Drawing for the job (mm, zero at the part's lowest x, y, z). A direction names the side the tool comes from. Give positions to 0.01 mm unless a question says otherwise; leave off trailing zeros. Loops run counter-clockwise (first coordinate to the right, second up) from the corner with the lowest first, then second, coordinate; pieces in that order, holes last.
1) Flat gauge pins, fed straight in: P1, Ø5.5, axis at x = 63.5, y = 24.003, coming from the +Z side (3 decimals); P2, Ø11.5, axis at x = 34.925, y = 16.002, coming from the +Z side; P3, Ø5, axis at x = 31.5, y = 18.5, coming from the -Z side; P4, Ø7.5, axis at x = 23.5, z = 8.5, coming from the +Y side (3 decimals). Where does each tip first touch, or does it go through?
2) Band-saw the part on D-D on x = 58.5. List the corners of the cut face in (y, z) (3 decimals).
3) Band-saw the part on C-C on y = 41. List the corners of the cut face in (x, z) (3 decimals), then the cut area to 3 significant figures.
4) 3-axis set-ups, long thin cutter, end or side, ignore diameter. For the marked faces 1 and 2: which of +Z, -Z, +X, -X, +Y, -Y reach the whole face in a straight line?
5) Band-saw the part on A-A on x = 6.35. List the corners of the cut face in (y, z) (3 decimals).
6) Band-saw the part on B-B on z = 6.35. List the corners of the cut face in (x, y) (3 decimals).
7) Wall check: line 1 (Y direction, x = 63.5, z = 2); line 2 (Y direction, x = 35, z = 11.5) (3 decimals). Give the ranges that are in metal, low to high.
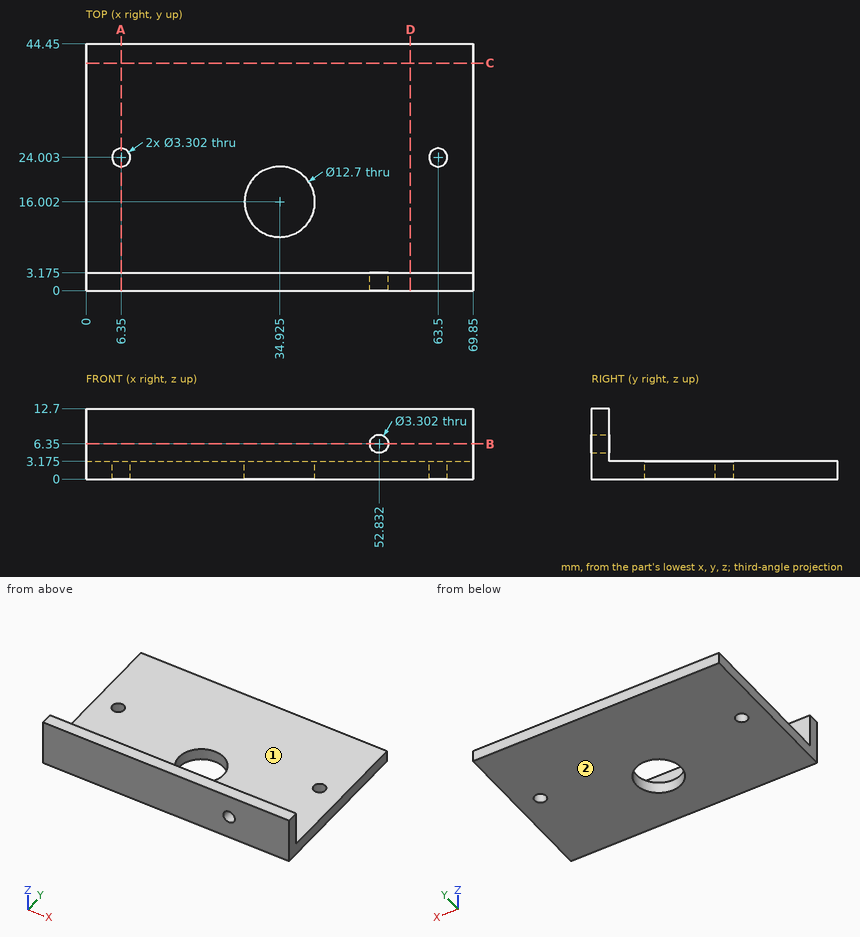
Findings below:
1. P1: stops at z = 3.175
1. P2: passes through
1. P3: stops at z = 0
1. P4: stops at y = 3.175
2. outline: (0, 0) - (44.45, 0) - (44.45, 3.175) - (3.175, 3.175) - (3.175, 12.7) - (0, 12.7) - close
3. outline: (0, 0) - (69.85, 0) - (69.85, 3.175) - (0, 3.175) - close
3. area: 222 mm2
4. face 1: +Z, +X, -X, +Y
4. face 2: -Z, +X, -X, +Y, -Y
5. outline: (0, 0) - (22.352, 0) - (22.352, 3.175) - (3.175, 3.175) - (3.175, 12.7) - (0, 12.7) - close; (25.654, 0) - (44.45, 0) - (44.45, 3.175) - (25.654, 3.175) - close
6. outline: (0, 0) - (51.181, 0) - (51.181, 3.175) - (0, 3.175) - close; (54.483, 0) - (69.85, 0) - (69.85, 3.175) - (54.483, 3.175) - close
7. line 1: y = 0 to 22.35, 25.65 to 44.45
7. line 2: y = 0 to 3.175
